Here's how the part is built. I have some questions about the finished solid (model axes, mm). A direction names the side the tool comes from. Coordinates: 2 decimals unless noted, no trailing zeros. Write each loop counter-clockwise with the first axis right and the second up, starting at its lowest first coordinate (ties: lowest second). Pieces come first, ordered by that corner, then holes. Notation, with made-up numbers: M 23.25,16.5 L 48.25,16.5 A13 cw 48.25,38.5 Z; hole C 40,47 d10. An arc over 180 degrees is marked long. Write each question's results on one line, items separated by ' | '. Start each with the question number.
from build123d import *

# Parameters (mm, degrees)
F0_W     = 82.024645
F0_H     = 77.41975
F1_DEPTH = 57.658
F2_R     = 23.894838
F3_DEPTH = 46.736
F4_R     = 19.003209
F5_DEPTH = 198.882


with BuildPart() as f1:
    # F0 (on Front) → F1 (new body)
    with BuildSketch(Plane.XZ):
        with Locations((1.43903, -1.151223)):
            Rectangle(F0_W, F0_H)
    extrude(amount=F1_DEPTH)

    # F2 (on face) → F3 (join)
    with BuildSketch(Plane.XZ.offset(57.658)):
        Circle(F2_R)
    extrude(amount=F3_DEPTH)

    # F4 (on face) → F5 (cut)
    with BuildSketch(Plane.XZ.offset(104.394)):
        Circle(F4_R)
    extrude(amount=-F5_DEPTH, mode=Mode.SUBTRACT)


solid = f1.part
1) I want a section at C-C, the plane y = -20.5. Write out the boundary of the cut face in (x, z).
2) We'd pull the mould along Z, two halves only. Please class faces 1 (the flat face through (-39.573, -28, -2)), 2 (the flat face through (1, -28, 37.559)), 3 (the cylindrical face through (-5.18, -80.699, -23.327)), 4 (the cylindrical face through (-15.08, -52.928, -11.563)): pulls with the +Z half, pulls with the -Z half, needs draft (parallel to the pull), parting line crosses it, or undercut.
3) For faces 5 (the flat face through (19, -57.658, 17)), 6 (the flat face through (10, 0, -18)), which set-ups out of +Z, -Z, +X, -X, +Y, -Y let a thin tool reach every point of the face, with its end or its side?
4) Please list where these lines run through material, in increasing order: line 1 (Z direction, x = 0, y = -72); line 2 (Z direction, x = 0, y = -37); line 3 (Y direction, x = 39, z = 33.5). Write a range as [from, to].
5) I want a section at A-A, the plane z = 0. Write out the boundary of the cut face in (x, y), then the cut area to 3 significant figures.
6) I want a section at D-D, the plane z = -30. Write out the boundary of the cut face in (x, y), then the cut area to 3 significant figures.
7) For pin 1 Ø3 at (x, y) = (-6.5, -61.5) entering from +Z; pin 2 Ø12 at (y, z) = (-82, 1) entering from -X, each with a flat end and sliding along its axis, tell me the tip position at first contact or that it passes through.
8) I want a section at B-B, the plane x = 0. Write out the boundary of the cut face in (y, z), then the cut area to 3 significant figures.
Output:
1) outline: M -39.57,-39.86 L 42.45,-39.86 L 42.45,37.56 L -39.57,37.56 Z; hole C 0,0 d38.01
2) face 1: needs draft | face 2: pulls with the +Z half | face 3: parting line crosses it | face 4: undercut
3) face 5: -Y | face 6: +Z, -Z, +X, -X, +Y
4) line 1: z = [-23.89, -19], [19, 23.89] | line 2: z = [-39.86, -19], [19, 37.56] | line 3: y = [-57.66, 0]
5) outline: M -39.57,-57.66 L -23.89,-57.66 L -23.89,-104.39 L -19,-104.39 L -19,0 L -39.57,0 Z; M 19,-104.39 L 23.89,-104.39 L 23.89,-57.66 L 42.45,-57.66 L 42.45,0 L 19,0 Z | area: 3,000 mm2
6) outline: M -39.57,-57.66 L 42.45,-57.66 L 42.45,0 L -39.57,0 Z | area: 4,730 mm2
7) pin 1: stops at z = 23.37 | pin 2: stops at x = -23.89
8) outline: M -104.39,-23.89 L -57.66,-23.89 L -57.66,-39.86 L 0,-39.86 L 0,-19 L -104.39,-19 Z; M -104.39,19 L 0,19 L 0,37.56 L -57.66,37.56 L -57.66,23.89 L -104.39,23.89 Z | area: 2,730 mm2
